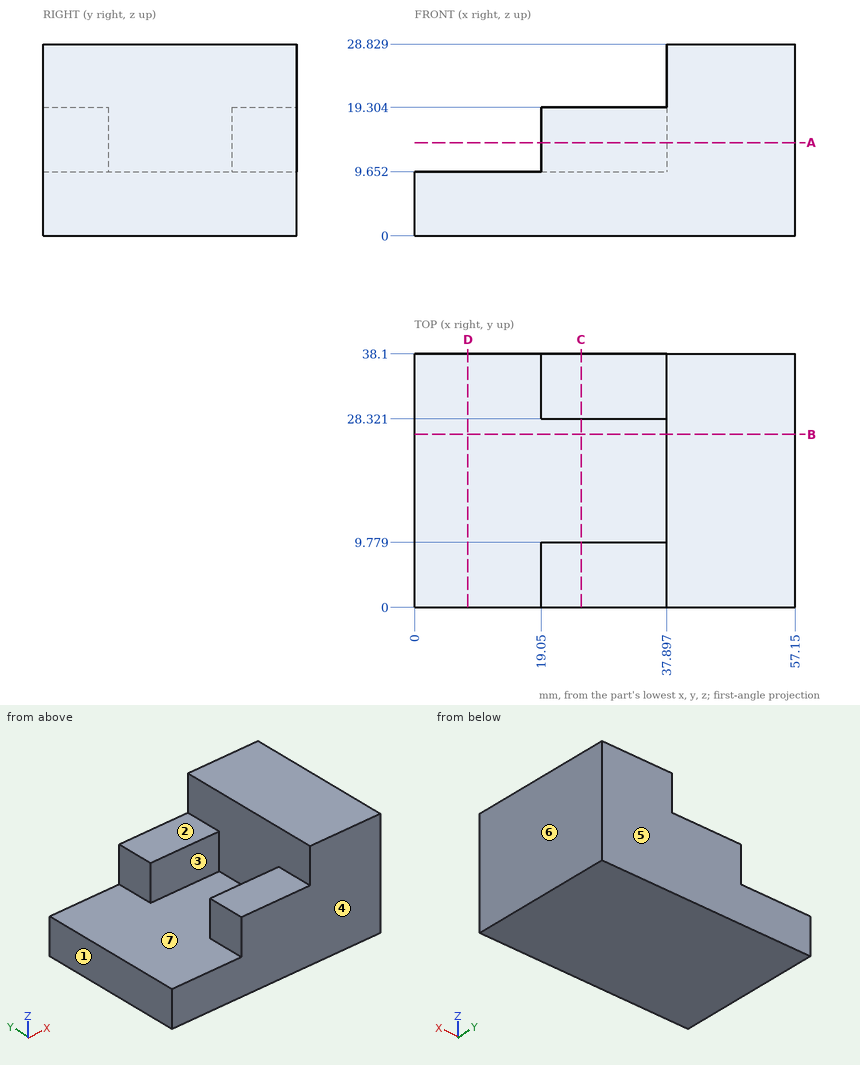
Verification items for this drawing (mm, ordinates from the low corner). A direction names the side the tool comes from. Coordinates: 2 decimals unless noted, no trailing zeros. Loops run counter-clockwise (first coordinate to the right, second up) from the corner with the lowest first, then second, coordinate; pieces in that order, holes last. Notation, with made-up numbers: (43, 55) -> (80, 55) arc R18 ccw to (80, 84) -> close; hole circle Ø9 at (6.5, 64). An arc over 180 degrees is marked (long way). Answer in a Markdown table with one row per item. Add a question column.
1. Depth check by flat-ended pin: P1, Ø11.5, axis at x = 15, y = 25, coming from the +Z side; P2, Ø1, axis at x = 49.5, y = 5, coming from the -Z side; P3, Ø3, axis at y = 6.5, z = 14, coming from the -X side; P4, Ø3, axis at y = 24, z = 15, coming from the -X side. Enter the tip coordinate at first touch or a pass-through.
2. Section check C-C, the plane x = 25. Enter the section's corners in (y, z).
3. Section check B-B, the plane y = 26. Enter the section's corners in (x, z).
4. Material ranges on probe 1 along Z at (x, y) = (37.5, 31.5); probe 2 along Z at (x, y) = (14.5, 8); probe 3 along X at (y, z) = (10, 18.75), recorded low to high. Write a range as [from, to].
5. Draft check along Y on the marked faces 4, 5, 6 and 7. Enter one of: +Y half, -Y half, draft (parallel to the pull), parting line (faces both ways), or undercut.
6. Section check D-D, the plane x = 8. Enter the section's corners in (y, z).
7. Section check A-A, the plane z = 14. Enter the section's corners in (x, y), then the cut area to 3 significant figures.
8. Access from +Z, -Z, +X, -X, +Y, -Y to the whole of each face (thin tool, end or side, straight path). Record for the marked faces 1, 2 and 3.
Derived:
| question | item | result |
|---|---|---|
| 1 | P1 | stops at z = 19.3 |
| 1 | P2 | stops at z = 0 |
| 1 | P3 | stops at x = 19.05 |
| 1 | P4 | stops at x = 37.9 |
| 2 | outline | (0, 0) -> (38.1, 0) -> (38.1, 19.3) -> (28.32, 19.3) -> (28.32, 9.65) -> (9.78, 9.65) -> (9.78, 19.3) -> (0, 19.3) -> close |
| 3 | outline | (0, 0) -> (57.15, 0) -> (57.15, 28.83) -> (37.9, 28.83) -> (37.9, 9.65) -> (0, 9.65) -> close |
| 4 | probe 1 | z = [0, 19.3] |
| 4 | probe 2 | z = [0, 9.65] |
| 4 | probe 3 | x = [37.9, 57.15] |
| 5 | face 4 | -Y half |
| 5 | face 5 | +Y half |
| 5 | face 6 | draft |
| 5 | face 7 | undercut |
| 6 | outline | (0, 0) -> (38.1, 0) -> (38.1, 9.65) -> (0, 9.65) -> close |
| 7 | outline | (19.05, 0) -> (57.15, 0) -> (57.15, 38.1) -> (19.05, 38.1) -> (19.05, 28.32) -> (37.9, 28.32) -> (37.9, 9.78) -> (19.05, 9.78) -> close |
| 7 | area | 1,100 mm² |
| 8 | face 1 | +Z, -Z, -X, +Y, -Y |
| 8 | face 2 | +Z, -X, +Y, -Y |
| 8 | face 3 | +Z, -X |
